Can you work these out from the model? Positions are in its coordinate system, mm. A direction names the side the tool comes from. Round coordinates to 2 decimals unless told otherwise and drop trailing zeros. Loops run counter-clockwise (first coordinate to the right, second up) from the corner with the lowest first, then second, coordinate; pieces in that order, holes last.
(1) If I drill on line 1 along Y through (x, z) = (28, 40); line 2 along Y through (x, z) = (-21.5, 17); line 3 along Z through (x, y) = (29, 4), over which ranges is the centre line in solid material (lowest first)?
(2) I want a section at B-B on z = 9. Give the number of separate pieces and of enclosed holes in the cut face, plus the area to 3 significant figures.
(3) I want a section at D-D on x = 19.05. Write out the boundary of the cut face in (y, z).
(4) Thinking about a two-plate mould opening in Y: for faces 4 (the face through (9.04, -0.04, 33.72)), 5 (the face through (26.201, 1.768, 14.079)), 6 (the face through (17, 7.764, 49)), which applies, released by +Y, released by -Y, zero draft, split by the parting line, or undercut?
(5) Which directions (+Z, -Z, +X, -X, +Y, -Y) give clear straight access to the entire face, cutting with the end or side of a thin tool? Please do faces 1 (the face through (30.08, 2.64, -0.79)), 2 (the face through (28, 15, 0.4)), 3 (the face through (-27.232, 10, 24)).
(6) Will these pins go through, and if not, where does the flat tip stop? pin 1 Ø2 at (x, y) = (0, 4.5) entering from -Z; pin 2 Ø4 at (x, y) = (14, 1.5) entering from +Z; pin 3 Ø3 at (x, y) = (1, 3) entering from +Z.
(7) I want a section at C-C on z = 59.5. Write out the boundary of the cut face in (x, y).
(8) I want a section at A-A on x = 40.8. Write out the boundary of the cut face in (y, z).
from build123d import *

# Parameters (mm, degrees)
F0_W     = 73.5817615905
F0_H     = 25.3
F0_R     = 3.45
F0_R_2   = 3.2
F0_R_3   = 2.95
F0_R_4   = 2.7
F0_R_5   = 2.45
F0_R_6   = 2.2
F0_R_7   = 1.95
F0_R_8   = 1.7
F0_R_9   = 1.45
F0_R_10  = 1.2
F0_R_11  = 0.95
F0_R_12  = 0.7
F0_R_13  = 3.7
F0_R_14  = 3.95
F0_R_15  = 4.2
F0_R_16  = 4.45
F0_R_17  = 4.7
F0_R_18  = 4.95
F0_R_19  = 5.2
F1_DEPTH = 80
F3_DEPTH = 0.4
F4_DEPTH = 10.7
F6_DEPTH = 25
F8_DEPTH = 1.6


with BuildPart() as f1:
    # F0 (on Top) → F1 (new body)
    with BuildSketch(Plane.XY):
        with Locations((9.5591192048, 9.7144579899)):
            Rectangle(F0_W, F0_H)
        with Locations((-15.2, 2.5144579899)):
            Circle(F0_R, mode=Mode.SUBTRACT)
        with Locations((-7.35, 2.5144579899)):
            Circle(F0_R_2, mode=Mode.SUBTRACT)
        with Locations((0, 2.5144579899)):
            Circle(F0_R_3, mode=Mode.SUBTRACT)
        with Locations((6.85, 2.5144579899)):
            Circle(F0_R_4, mode=Mode.SUBTRACT)
        with Locations((13.2, 2.5144579899)):
            Circle(F0_R_5, mode=Mode.SUBTRACT)
        with Locations((19.05, 2.5144579899)):
            Circle(F0_R_6, mode=Mode.SUBTRACT)
        with Locations((24.4, 2.5144579899)):
            Circle(F0_R_7, mode=Mode.SUBTRACT)
        with Locations((29.25, 2.5144579899)):
            Circle(F0_R_8, mode=Mode.SUBTRACT)
        with Locations((33.6, 2.5144579899)):
            Circle(F0_R_9, mode=Mode.SUBTRACT)
        with Locations((37.45, 2.5144579899)):
            Circle(F0_R_10, mode=Mode.SUBTRACT)
        with Locations((40.8, 2.5144579899)):
            Circle(F0_R_11, mode=Mode.SUBTRACT)
        with Locations((43.65, 2.5144579899)):
            Circle(F0_R_12, mode=Mode.SUBTRACT)
        with Locations((-21.5317615905, 15.1644579899)):
            Circle(F0_R_13, mode=Mode.SUBTRACT)
        with Locations((-12.6817615905, 15.1644579899)):
            Circle(F0_R_14, mode=Mode.SUBTRACT)
        with Locations((-3.3317615905, 15.1644579899)):
            Circle(F0_R_15, mode=Mode.SUBTRACT)
        with Locations((6.5182384095, 15.1644579899)):
            Circle(F0_R_16, mode=Mode.SUBTRACT)
        with Locations((16.8682384095, 15.1644579899)):
            Circle(F0_R_17, mode=Mode.SUBTRACT)
        with Locations((27.7182384095, 15.1644579899)):
            Circle(F0_R_18, mode=Mode.SUBTRACT)
        with Locations((39.0682384095, 15.1644579899)):
            Circle(F0_R_19, mode=Mode.SUBTRACT)
    extrude(amount=F1_DEPTH)

    # F2 (on face) → F4 (cut)
    with BuildSketch(Plane.XZ.offset(2.9355420101)):
        Polygon((-27.2317615905, 80), (-27.2317615905, 49), (46.35, 18), (46.35, 80), align=None)
    extrude(amount=-F4_DEPTH, mode=Mode.SUBTRACT)

    # F5 (on face) → F6 (cut)
    with BuildSketch(Plane(origin=(0, 22.3644579899, 0), x_dir=(-1, 0, 0), z_dir=(0, 1, 0))):
        Polygon((-46.35, 80), (27.2317615905, 49), (27.2317615905, 80), align=None)
    extrude(amount=-F6_DEPTH, mode=Mode.SUBTRACT)



with BuildPart() as f3:
    # F0 (on Top) → F3 (new body)
    with BuildSketch(Plane.XY):
        with Locations((9.5591192048, 9.7144579899)):
            Rectangle(F0_W, F0_H)
        with Locations((-15.2, 2.5144579899)):
            Circle(F0_R, mode=Mode.SUBTRACT)
        with Locations((-7.35, 2.5144579899)):
            Circle(F0_R_2, mode=Mode.SUBTRACT)
        with Locations((0, 2.5144579899)):
            Circle(F0_R_3, mode=Mode.SUBTRACT)
        with Locations((6.85, 2.5144579899)):
            Circle(F0_R_4, mode=Mode.SUBTRACT)
        with Locations((13.2, 2.5144579899)):
            Circle(F0_R_5, mode=Mode.SUBTRACT)
        with Locations((19.05, 2.5144579899)):
            Circle(F0_R_6, mode=Mode.SUBTRACT)
        with Locations((24.4, 2.5144579899)):
            Circle(F0_R_7, mode=Mode.SUBTRACT)
        with Locations((29.25, 2.5144579899)):
            Circle(F0_R_8, mode=Mode.SUBTRACT)
        with Locations((33.6, 2.5144579899)):
            Circle(F0_R_9, mode=Mode.SUBTRACT)
        with Locations((37.45, 2.5144579899)):
            Circle(F0_R_10, mode=Mode.SUBTRACT)
        with Locations((40.8, 2.5144579899)):
            Circle(F0_R_11, mode=Mode.SUBTRACT)
        with Locations((43.65, 2.5144579899)):
            Circle(F0_R_12, mode=Mode.SUBTRACT)
        with Locations((-21.5317615905, 15.1644579899)):
            Circle(F0_R_13, mode=Mode.SUBTRACT)
        with Locations((-12.6817615905, 15.1644579899)):
            Circle(F0_R_14, mode=Mode.SUBTRACT)
        with Locations((-3.3317615905, 15.1644579899)):
            Circle(F0_R_15, mode=Mode.SUBTRACT)
        with Locations((6.5182384095, 15.1644579899)):
            Circle(F0_R_16, mode=Mode.SUBTRACT)
        with Locations((16.8682384095, 15.1644579899)):
            Circle(F0_R_17, mode=Mode.SUBTRACT)
        with Locations((27.7182384095, 15.1644579899)):
            Circle(F0_R_18, mode=Mode.SUBTRACT)
        with Locations((39.0682384095, 15.1644579899)):
            Circle(F0_R_19, mode=Mode.SUBTRACT)
        with Locations((39.0682384095, 15.1644579899)):
            Circle(F0_R_19)
        with Locations((27.7182384095, 15.1644579899)):
            Circle(F0_R_18)
        with Locations((16.8682384095, 15.1644579899)):
            Circle(F0_R_17)
        with Locations((6.5182384095, 15.1644579899)):
            Circle(F0_R_16)
        with Locations((-3.3317615905, 15.1644579899)):
            Circle(F0_R_15)
        with Locations((-12.6817615905, 15.1644579899)):
            Circle(F0_R_14)
        with Locations((-21.5317615905, 15.1644579899)):
            Circle(F0_R_13)
        with Locations((-15.2, 2.5144579899)):
            Circle(F0_R)
        with Locations((-7.35, 2.5144579899)):
            Circle(F0_R_2)
        with Locations((0, 2.5144579899)):
            Circle(F0_R_3)
        with Locations((6.85, 2.5144579899)):
            Circle(F0_R_4)
        with Locations((13.2, 2.5144579899)):
            Circle(F0_R_5)
        with Locations((19.05, 2.5144579899)):
            Circle(F0_R_6)
        with Locations((24.4, 2.5144579899)):
            Circle(F0_R_7)
        with Locations((29.25, 2.5144579899)):
            Circle(F0_R_8)
        with Locations((33.6, 2.5144579899)):
            Circle(F0_R_9)
        with Locations((37.45, 2.5144579899)):
            Circle(F0_R_10)
        with Locations((40.8, 2.5144579899)):
            Circle(F0_R_11)
        with Locations((43.65, 2.5144579899)):
            Circle(F0_R_12)
    extrude(amount=F3_DEPTH)


with BuildPart() as f1_1:
    add(f1.part)

    add(f3.part)  # F8 merges F3
    # F7 (on face) → F8 (join)
    with BuildSketch(Plane(origin=(0, 0, 0), x_dir=(1, 0, 0), z_dir=(0, 0, -1))):
        with BuildLine():
            Line((-19.1681346587, -3.8992594928), (-27.2317615905, -3.8992594928))
            Line((-27.2317615905, -3.8992594928), (-27.2317615905, -14.6005405113))
            Line((-27.2317615905, -14.6005405113), (-19.1681346587, -14.6005405113))
            ThreePointArc((-19.1681346587, -14.6005405113), (-14.9681346587, -10.4005405113), (-10.7681346587, -14.6005405113))
            Line((-10.7681346587, -14.6005405113), (-6.904507727, -14.6005405113))
            ThreePointArc((-6.904507727, -14.6005405113), (-2.704507727, -10.4005405113), (1.495492273, -14.6005405113))
            Line((1.495492273, -14.6005405113), (5.3591192048, -14.6005405113))
            ThreePointArc((5.3591192048, -14.6005405113), (9.5591192048, -10.4005405113), (13.7591192048, -14.6005405113))
            Line((13.7591192048, -14.6005405113), (17.6227461365, -14.6005405113))
            ThreePointArc((17.6227461365, -14.6005405113), (21.8227461365, -10.4005405113), (26.0227461365, -14.6005405113))
            Line((26.0227461365, -14.6005405113), (29.8863730683, -14.6005405113))
            ThreePointArc((29.8863730683, -14.6005405113), (34.0863730683, -10.4005405113), (38.2863730683, -14.6005405113))
            Line((38.2863730683, -14.6005405113), (46.35, -14.6005405113))
            Line((46.35, -14.6005405113), (46.35, -3.8992594928))
            Line((46.35, -3.8992594928), (38.2863730683, -3.8992594928))
            ThreePointArc((38.2863730683, -3.8992594928), (34.0863730683, -8.0992594928), (29.8863730683, -3.8992594928))
            Line((29.8863730683, -3.8992594928), (26.0227461365, -3.8992594928))
            ThreePointArc((26.0227461365, -3.8992594928), (21.8227461365, -8.0992594928), (17.6227461365, -3.8992594928))
            Line((17.6227461365, -3.8992594928), (13.7591192048, -3.8992594928))
            ThreePointArc((13.7591192048, -3.8992594928), (9.5591192048, -8.0992594928), (5.3591192048, -3.8992594928))
            Line((5.3591192048, -3.8992594928), (1.495492273, -3.8992594928))
            ThreePointArc((1.495492273, -3.8992594928), (-2.704507727, -8.0992594928), (-6.904507727, -3.8992594928))
            Line((-6.904507727, -3.8992594928), (-10.7681346587, -3.8992594928))
            ThreePointArc((-10.7681346587, -3.8992594928), (-14.9681346587, -8.0992594928), (-19.1681346587, -3.8992594928))
        make_face()
        with BuildLine():
            Line((46.35, 2.9355420101), (-27.2317615905, 2.9355420101))
            Line((-27.2317615905, 2.9355420101), (-27.2317615905, -3.8992594928))
            Line((-27.2317615905, -3.8992594928), (-19.1681346587, -3.8992594928))
            ThreePointArc((-19.1681346587, -3.8992594928), (-14.9681346587, 0.3007405072), (-10.7681346587, -3.8992594928))
            Line((-10.7681346587, -3.8992594928), (-6.904507727, -3.8992594928))
            ThreePointArc((-6.904507727, -3.8992594928), (-2.704507727, 0.3007405072), (1.495492273, -3.8992594928))
            Line((1.495492273, -3.8992594928), (5.3591192048, -3.8992594928))
            ThreePointArc((5.3591192048, -3.8992594928), (9.5591192048, 0.3007405072), (13.7591192048, -3.8992594928))
            Line((13.7591192048, -3.8992594928), (17.6227461365, -3.8992594928))
            ThreePointArc((17.6227461365, -3.8992594928), (21.8227461365, 0.3007405072), (26.0227461365, -3.8992594928))
            Line((26.0227461365, -3.8992594928), (29.8863730683, -3.8992594928))
            ThreePointArc((29.8863730683, -3.8992594928), (34.0863730683, 0.3007405072), (38.2863730683, -3.8992594928))
            Line((38.2863730683, -3.8992594928), (46.35, -3.8992594928))
            Line((46.35, -3.8992594928), (46.35, 2.9355420101))
        make_face()
        with BuildLine():
            Line((-19.1681346587, -14.6005405113), (-27.2317615905, -14.6005405113))
            Line((-27.2317615905, -14.6005405113), (-27.2317615905, -22.3644579899))
            Line((-27.2317615905, -22.3644579899), (46.35, -22.3644579899))
            Line((46.35, -22.3644579899), (46.35, -14.6005405113))
            Line((46.35, -14.6005405113), (38.2863730683, -14.6005405113))
            ThreePointArc((38.2863730683, -14.6005405113), (34.0863730683, -18.8005405113), (29.8863730683, -14.6005405113))
            Line((29.8863730683, -14.6005405113), (26.0227461365, -14.6005405113))
            ThreePointArc((26.0227461365, -14.6005405113), (21.8227461365, -18.8005405113), (17.6227461365, -14.6005405113))
            Line((17.6227461365, -14.6005405113), (13.7591192048, -14.6005405113))
            ThreePointArc((13.7591192048, -14.6005405113), (9.5591192048, -18.8005405113), (5.3591192048, -14.6005405113))
            Line((5.3591192048, -14.6005405113), (1.495492273, -14.6005405113))
            ThreePointArc((1.495492273, -14.6005405113), (-2.704507727, -18.8005405113), (-6.904507727, -14.6005405113))
            Line((-6.904507727, -14.6005405113), (-10.7681346587, -14.6005405113))
            ThreePointArc((-10.7681346587, -14.6005405113), (-14.9681346587, -18.8005405113), (-19.1681346587, -14.6005405113))
        make_face()
    extrude(amount=F8_DEPTH)


solid = f1_1.part
Filled sheet:
1. line 1: y = 7.76 to 10.22, 20.11 to 22.36
1. line 2: y = -2.94 to 11.46, 18.86 to 22.36
1. line 3: z = -1.6 to 0.4
2. separate pieces: 1
2. enclosed holes: 19
2. area: 1,230 mm2
3. outline: (-2.94, -1.6) - (0.74, -1.6) - (0.74, 0) - (7.05, 0) - (7.05, -1.6) - (11.45, -1.6) - (11.45, 0) - (17.76, 0) - (17.76, -1.6) - (22.36, -1.6) - (22.36, 68.5) - (19.33, 68.5) - (19.33, 0.4) - (11, 0.4) - (11, 68.5) - (7.76, 68.5) - (7.76, 29.5) - (4.71, 29.5) - (4.71, 0.4) - (0.31, 0.4) - (0.31, 29.5) - (-2.94, 29.5) - close
4. face 4: zero draft
4. face 5: undercut
4. face 6: released by -Y
5. face 1: -Z
5. face 2: +Z
5. face 3: +Z, -Z, -X, +Y, -Y
6. pin 1: stops at z = 0
6. pin 2: stops at z = 32.26
6. pin 3: stops at z = 0.4
7. outline: (-2.31, 7.76) - (46.35, 7.76) - (46.35, 22.36) - (-2.31, 22.36) - (-2.31, 19.24) arc R4.2 cw to (-2.31, 11.09) - close; hole circle Ø8.9 at (6.52, 15.16); hole circle Ø9.4 at (16.87, 15.16); hole circle Ø9.9 at (27.72, 15.16); hole circle Ø10.4 at (39.07, 15.16)
8. outline: (-2.94, -1.6) - (22.36, -1.6) - (22.36, 77.66) - (20.07, 77.66) - (20.07, 0.4) - (10.26, 0.4) - (10.26, 77.66) - (7.76, 77.66) - (7.76, 20.34) - (3.46, 20.34) - (3.46, 0.4) - (1.56, 0.4) - (1.56, 20.34) - (-2.94, 20.34) - close
